from build123d import *

# Parameters (mm, degrees)
SKETCH1_W           = 40
SKETCH1_H           = 85
BOSS_EXTRUDE1_DEPTH = 75
SKETCH3_OUTSIDE_W   = 66.042
SKETCH3_OUTSIDE_H   = 111.042
SKETCH3_OUTSIDE_W_2 = 40
SKETCH3_OUTSIDE_H_2 = 85
SKETCH3_OUTSIDE_W_3 = 30
SKETCH3_OUTSIDE_H_3 = 75
CUT_EXTRUDE2_DEPTH  = 70
SKETCH4_W           = 35
SKETCH4_H           = 85
CUT_EXTRUDE3_DEPTH  = 30
FILLET1_R           = 10
SKETCH5_R           = 2.5
CUT_EXTRUDE4_DEPTH  = 30
CHAMFER1_SIZE       = 1
CUT_EXTRUDE5_DEPTH  = 30
FILLET2_R           = 1
FILLET3_R           = 10
SKETCH7_W           = 14
SKETCH7_H           = 53
CUT_EXTRUDE6_DEPTH  = 30
FILLET4_R           = 1
CUT_EXTRUDE7_DEPTH  = 30
FILLET5_R           = 10
SKETCH9_R           = 2.5
CUT_EXTRUDE8_DEPTH  = 30
CHAMFER2_SIZE       = 1
SKETCH10_W          = 20
SKETCH10_H          = 25
CUT_EXTRUDE9_DEPTH  = 130
FILLET6_R           = 1
FILLET7_R           = 1
SKETCH12_W          = 99.145482585
SKETCH12_H          = 91.596568109
CUT_EXTRUDE11_DEPTH = 2.5
SKETCH13_W          = 51.22831634
SKETCH13_H          = 105.793314496
CUT_EXTRUDE12_DEPTH = 2.5
SKETCH14_W          = 73
SKETCH14_H          = 70.039653543
CUT_EXTRUDE13_DEPTH = 2.5


# Some blends are built 0.0001 mm under size
with BuildPart() as part:
    # Sketch1 → Boss-Extrude1 (new body)
    with BuildSketch(Plane(origin=(0, 0, 0), x_dir=(1, 0, 0), z_dir=(0, 1, 0))):
        with Locations((-11.153846154, 11.538461538)):
            Rectangle(SKETCH1_W, SKETCH1_H)
    extrude(amount=BOSS_EXTRUDE1_DEPTH)

    # Sketch3 outside → Cut-Extrude2 (cut)
    # profile 1 of 2: a face of its own
    with BuildSketch(Plane(origin=(0, 75, 0), x_dir=(1, 0, 0), z_dir=(0, 1, 0))):
        with Locations((-11.154, 11.538)):
            Rectangle(SKETCH3_OUTSIDE_W, SKETCH3_OUTSIDE_H)
        with Locations((-11.153846154, 11.538461538)):
            Rectangle(SKETCH3_OUTSIDE_W_2, SKETCH3_OUTSIDE_H_2, mode=Mode.SUBTRACT)
    # profile 2 of 2: a face of its own
    with BuildSketch(Plane(origin=(0, 75, 0), x_dir=(1, 0, 0), z_dir=(0, 1, 0))):
        with Locations((-11.153846154, 11.538461538)):
            Rectangle(SKETCH3_OUTSIDE_W_3, SKETCH3_OUTSIDE_H_3)
    extrude(amount=-CUT_EXTRUDE2_DEPTH, mode=Mode.SUBTRACT)

    # Sketch4 → Cut-Extrude3 (cut)
    with BuildSketch(Plane(origin=(0, 75, 0), x_dir=(1, 0, 0), z_dir=(0, 1, 0))):
        with Locations((-8.653846154, 11.538461538)):
            Rectangle(SKETCH4_W, SKETCH4_H)
    extrude(amount=-CUT_EXTRUDE3_DEPTH, mode=Mode.SUBTRACT)

    # Fillet1
    fillet1_edges = [part.edges().sort_by_distance(p)[0] for p in [
        (-28.653846154, 75, -54.038461538),
        (-28.653846154, 75, 30.961538462),
    ]]
    fillet(fillet1_edges, radius=FILLET1_R)

    # Sketch5 → Cut-Extrude4 (cut)
    with BuildSketch(Plane(origin=(-26.153846154, 0, 0), x_dir=(0, 0, -1), z_dir=(1, 0, 0))):
        with Locations((-20.961538462, 65)):
            Circle(SKETCH5_R)
        with Locations((44.038461538, 65)):
            Circle(SKETCH5_R)
    extrude(amount=-CUT_EXTRUDE4_DEPTH, mode=Mode.SUBTRACT)

    # Chamfer1
    chamfer1_edges = [part.edges().sort_by_distance(p)[0] for p in [
        (-26.153846154, 65, 23.461538462),
        (-26.153846154, 65, -41.538461538),
    ]]
    chamfer(chamfer1_edges, length=CHAMFER1_SIZE)

    # Sketch6 → Cut-Extrude5 (cut)
    with BuildSketch(Plane(origin=(8.846153846, 0, 0), x_dir=(0, 0, -1), z_dir=(1, 0, 0))):
        with BuildLine():
            Line((-15.961538462, 45), (39.038461538, 45))
            Line((39.038461538, 45), (39.038461538, 40))
            ThreePointArc((39.038461538, 40), (36.10952935, 32.928932188), (29.038461538, 30))
            Line((29.038461538, 30), (-5.961538462, 30))
            ThreePointArc((-5.961538462, 30), (-13.032606273, 32.928932188), (-15.961538462, 40))
            Line((-15.961538462, 40), (-15.961538462, 45))
        make_face()
    extrude(amount=-CUT_EXTRUDE5_DEPTH, mode=Mode.SUBTRACT)

    # Fillet2
    fillet2_edges = [part.edges().sort_by_distance(p)[0] for p in [
        (-11.153846154, 5, 25.961538462),
        (3.846153846, 25, 25.961538462),
        (-26.153846154, 5, -11.538461538),
        (-26.153846154, 25, 25.961538462),
        (-11.153846154, 5, -49.038461538),
        (-26.153846154, 25, -49.038461538),
        (3.846153846, 5, -11.538461538),
        (3.846153846, 25, -49.038461538),
    ]]
    fillet(fillet2_edges, radius=FILLET2_R)

    # Fillet3
    # the kernel refuses this fillet: 10 mm, written as the material it takes off along each edge
    with BuildSketch(Plane(origin=(32.258445674, 45, 15.961538462), x_dir=(0, -0.9991049126334702, -0.04230098759681175), z_dir=(-1, 0, 0))) as fillet3_piece_1:
        with BuildLine():
            CenterArc((9.5949039, 9.779544188), FILLET3_R, 182.424391449, 75.522487814)
            Line((-0.396145226, 9.356534312), (-1.395250139, 9.314233325))
            Line((-1.395250139, 9.314233325), (-0.999104913, -0.042300988))
            Line((-0.999104913, -0.042300988), (0.042300988, -0.999104913))
            ThreePointArc((0.042300988, -0.999104913), (5.037825551, -0.787599975), (7.297900696, -0.977954419))
            Line((7.297900696, -0.977954419), (7.506719169, 0))
        make_face()
    extrude(amount=51.824583655, mode=Mode.SUBTRACT)
    with BuildSketch(Plane(origin=(32.258445674, 45, -39.038461538), x_dir=(0, -0.9991049126334705, 0.04230098759681053), z_dir=(-1, 0, 0))) as fillet3_piece_2:
        with BuildLine():
            CenterArc((9.5949039, -9.779544188), FILLET3_R, 102.053120737, 75.522487814)
            Line((-0.396145226, -9.356534312), (-1.395250139, -9.314233325))
            Line((-1.395250139, -9.314233325), (-0.999104913, 0.042300988))
            Line((-0.999104913, 0.042300988), (0.042300988, 0.999104913))
            ThreePointArc((0.042300988, 0.999104913), (5.037825551, 0.787599975), (7.297900696, 0.977954419))
            Line((7.297900696, 0.977954419), (7.506719169, 0))
        make_face()
    extrude(amount=51.824583655, mode=Mode.SUBTRACT)

    # Sketch7 → Cut-Extrude6 (cut)
    with BuildSketch(Plane(origin=(0, 5, 0), x_dir=(1, 0, 0), z_dir=(0, 1, 0))):
        with Locations((-11.153846154, 11.538461538)):
            Rectangle(SKETCH7_W, SKETCH7_H)
    extrude(amount=-CUT_EXTRUDE6_DEPTH, mode=Mode.SUBTRACT)

    # Fillet4
    fillet4_edges = [part.edges().sort_by_distance(p)[0] for p in [
        (-18.153846154, 5, -11.538461538),
        (-11.153846154, 5, 14.961538462),
        (-4.153846154, 5, -11.538461538),
        (-11.153846154, 5, -38.038461538),
    ]]
    fillet(fillet4_edges, radius=FILLET4_R)

    # Sketch8 → Cut-Extrude7 (cut)
    with BuildSketch(Plane(origin=(-26.153846154, 0, 0), x_dir=(0, 0, -1), z_dir=(1, 0, 0))):
        with BuildLine():
            Line((-10.961538462, 75), (34.038461538, 75))
            Line((34.038461538, 75), (34.038461538, 55))
            ThreePointArc((34.038461538, 55), (31.10952935, 47.928932188), (24.038461538, 45))
            Line((24.038461538, 45), (-0.961538462, 45))
            ThreePointArc((-0.961538462, 45), (-8.032606273, 47.928932188), (-10.961538462, 55))
            Line((-10.961538462, 55), (-10.961538462, 75))
        make_face()
    extrude(amount=-CUT_EXTRUDE7_DEPTH, mode=Mode.SUBTRACT)

    # Fillet5
    fillet5_edges = [part.edges().sort_by_distance(p)[0] for p in [
        (-28.653846154, 75, -34.038461538),
        (-28.653846154, 75, 10.961538462),
    ]]
    fillet(fillet5_edges, radius=FILLET5_R - 0.0001)  # a hair under: the kernel refuses the full size

    # Sketch9 → Cut-Extrude8 (cut)
    with BuildSketch(Plane(origin=(-26.153846154, 0, 0), x_dir=(0, 0, -1), z_dir=(1, 0, 0))):
        with Locations((11.538461538, 35)):
            Circle(SKETCH9_R)
    extrude(amount=-CUT_EXTRUDE8_DEPTH, mode=Mode.SUBTRACT)

    # Chamfer2
    chamfer2_edges = [part.edges().sort_by_distance(p)[0] for p in [
        (-26.153846154, 35, -9.038461538),
    ]]
    chamfer(chamfer2_edges, length=CHAMFER2_SIZE)

    # Sketch10 → Cut-Extrude9 (cut)
    with BuildSketch(Plane.XY.offset(30.961538462)):
        with Locations((-11.153846154, 22.5)):
            Rectangle(SKETCH10_W, SKETCH10_H)
    extrude(amount=-CUT_EXTRUDE9_DEPTH, mode=Mode.SUBTRACT)

    # Fillet6
    fillet6_edges = [part.edges().sort_by_distance(p)[0] for p in [
        (-21.153846154, 22.5, 25.961538462),
        (-11.153846154, 35, 25.961538462),
        (-1.153846154, 22.5, 25.961538462),
        (-11.153846154, 10, 25.961538462),
        (-21.153846154, 22.5, 30.961538462),
        (-11.153846154, 10, 30.961538462),
        (-1.153846154, 22.5, 30.961538462),
        (-11.153846154, 35, 30.961538462),
    ]]
    fillet(fillet6_edges, radius=FILLET6_R)

    # Fillet7
    fillet7_edges = [part.edges().sort_by_distance(p)[0] for p in [
        (-11.153846154, 10, -49.038461538),
        (-1.153846154, 22.5, -49.038461538),
        (-11.153846154, 35, -49.038461538),
        (-21.153846154, 22.5, -49.038461538),
        (-21.153846154, 22.5, -54.038461538),
        (-11.153846154, 35, -54.038461538),
        (-1.153846154, 22.5, -54.038461538),
        (-11.153846154, 10, -54.038461538),
    ]]
    fillet(fillet7_edges, radius=FILLET7_R)

    # Sketch12 → Cut-Extrude11 (cut)
    with BuildSketch(Plane.ZY.offset(31.153846154)):
        with Locations((-8.86612538, 45.798284055)):
            Rectangle(SKETCH12_W, SKETCH12_H)
    extrude(amount=-CUT_EXTRUDE11_DEPTH, mode=Mode.SUBTRACT)

    # Sketch13 → Cut-Extrude12 (cut)
    with BuildSketch(Plane.XZ):
        with Locations((-8.23266401, -21.935118786)):
            Rectangle(SKETCH13_W, SKETCH13_H)
    extrude(amount=-CUT_EXTRUDE12_DEPTH, mode=Mode.SUBTRACT)

    # Sketch14 → Cut-Extrude13 (cut)
    with BuildSketch(Plane.ZY.offset(-3.846153846)):
        with Locations((-11.538461538, 41.019826772)):
            Rectangle(SKETCH14_W, SKETCH14_H)
    extrude(amount=-CUT_EXTRUDE13_DEPTH, mode=Mode.SUBTRACT)


solid = part.part
Work out the finished part from the listing and answer in its coordinate system (mm). A direction names the side the tool comes from. Give positions to 0.01 mm unless a question says otherwise; leave off trailing zeros. Loops run counter-clockwise (first coordinate to the right, second up) from the corner with the lowest first, then second, coordinate; pieces in that order, holes last. Notation, with made-up numbers: (19.5, -8) -> (73.5, -8) arc R24 cw to (73.5, 3) -> close; hole circle Ø10 at (82, 48.25). An arc over 180 degrees is marked (long way). Use a Markdown table: item, result. Add a question column.
1. Section C-C on x = -9.5 is taken. State how many separate pieces and enclosed holes the cut face has, and give its area (3 significant figures).
2. For faces 1 (the flat face through (-27, 60, -34.038)), 2 (the flat face through (8, 30, -12)), 3 (the flat face through (-11, 35, 28)), 4 (the flat face through (6.346, 21, -12)), determine the directions among +Z, -Z, +X, -X, +Y, -Y from which every point of the face is accessible in a straight line to the end or side of a thin tool.
3. Section B-B on z = -5 is taken. Determine the outline of the cut face in (x, y), and give its area (3 significant figures).
4. Find the intervals of material crossed by probe 1 along Z at (x, y) = (4, 38); probe 2 along X at (y, z) = (11, -15.5); probe 3 along Z at (x, y) = (7, 44), in increasing order.
5. Section D-D on y = 60 is taken. Determine the outline of the cut face in (x, z), and give its area (3 significant figures).
6. Determine the mould class of faces 5 (the cylindrical face through (-27.89, 35.11, -9.04)), 6 (the flat face through (-28.654, 31, -12)), 7 (the flat face through (5, 25, 24.962)) for opening direction X: released by +X, released by -X, zero draft, split by the parting line, or undercut.
7. Flat-ended cylindrical pins translate along their axes: pin 1 Ø3 at (x, z) = (-27.5, -16.5) entering from +Y; pin 2 Ø3 at (x, z) = (4.5, -24.5) entering from +Y; pin 3 Ø2 at (x, z) = (7.5, -6) entering from +Y. Find the tip coordinate at first contact, or state that the pin passes through.
Results below:
| question | item | result |
|---|---|---|
| 1 | separate pieces | 4 |
| 1 | enclosed holes | 0 |
| 1 | area | 228 mm^2 |
| 2 | face 1 | +X, -X, +Y |
| 2 | face 2 | +X, +Y |
| 2 | face 3 | +Z, -Z |
| 2 | face 4 | +Y |
| 3 | outline | (-28.65, 2.5) -> (-18.15, 2.5) -> (-18.15, 4) arc R1 ccw to (-19.15, 5) -> (-25.15, 5) arc R1 cw to (-26.15, 6) -> (-26.15, 45) -> (-28.65, 45) -> close; (-4.15, 2.5) -> (8.85, 2.5) -> (8.85, 30) -> (6.35, 30) -> (6.35, 6) -> (3.85, 6) arc R1 cw to (2.85, 5) -> (-3.15, 5) arc R1 ccw to (-4.15, 4) -> close |
| 3 | area | 224 mm^2 |
| 4 | probe 1 | z = -54.04 to -48.04, 24.96 to 30.96 |
| 4 | probe 2 | x = -28.65 to -26.15, 6.35 to 8.85 |
| 4 | probe 3 | z = -54.04 to -44.04, 20.97 to 30.96 |
| 5 | outline | (-28.65, -54.04) -> (-26.15, -54.04) -> (-26.15, -34.04) -> (-28.65, -34.04) -> close; (-28.65, 10.96) -> (-26.15, 10.96) -> (-26.15, 30.96) -> (-28.65, 30.96) -> close |
| 5 | area | 100 mm^2 |
| 6 | face 5 | zero draft |
| 6 | face 6 | released by -X |
| 6 | face 7 | undercut |
| 7 | pin 1 | stops at y = 45 |
| 7 | pin 2 | stops at y = 6 |
| 7 | pin 3 | stops at y = 30 |
